Geometry: final body of the model. Coordinates: model frame, mm. A direction names the side the tool comes from. Give positions to 0.01 mm unless a question says otherwise; leave off trailing zeros. Write each loop counter-clockwise with the first axis right and the second up, starting at its lowest first coordinate (ties: lowest second). Pieces come first, ordered by that corner, then holes. Notation, with made-up numbers: (60.25, 45) -> (72.25, 45) arc R34 cw to (72.25, 81) -> close; hole circle Ø10 at (33.25, 53). An arc over 180 degrees is marked (long way). Answer as a JSON object with one key per item and string values.
from build123d import *

# Parameters (mm, degrees)
SKETCH001_W     = 40
SKETCH001_H     = 13.5
PAD_DEPTH       = 1
FILLET_R        = 2
SKETCH002_R     = 0.8
POCKET_DEPTH    = 85.45809
SKETCH_W        = 20
SKETCH_H        = 1.5
PAD001_DEPTH    = 3
SKETCH003_W     = 44
SKETCH003_H     = 1.5
PAD002_DEPTH    = 10
SKETCH005_R     = 2
POCKET001_DEPTH = 98.464305
PAD003_DEPTH    = 20


with BuildPart() as part:
    # Sketch001 → Pad (new body)
    with BuildSketch(Plane.XY):
        Rectangle(SKETCH001_W, SKETCH001_H)
    extrude(amount=PAD_DEPTH)

    # Fillet
    fillet_edges = [part.edges().sort_by_distance(p)[0] for p in [
        (20, 6.75, 0.5),
        (20, -6.75, 0.5),
        (-20, -6.75, 0.5),
        (-20, 6.75, 0.5),
    ]]
    fillet(fillet_edges, radius=FILLET_R)

    # Sketch002 (on Face5 of Fillet) → Pocket (cut, through all)
    with BuildSketch(Plane.XY.offset(1)):
        with Locations((-11, 5.75)):
            Circle(SKETCH002_R)
    pocket = extrude(amount=-POCKET_DEPTH, mode=Mode.SUBTRACT)

    # Mirrored: Pocket across Sketch002 V_Axis
    add(pocket.mirror(Plane(origin=(0, 0, 1), x_dir=(0, 0, 1), z_dir=(1, 0, 0))), mode=Mode.SUBTRACT)

    # Sketch (on Face5 of Mirrored) → Pad001 (join)
    with BuildSketch(Plane.XY.offset(1)):
        with Locations((0, -5.25)):
            Rectangle(SKETCH_W, SKETCH_H)
    extrude(amount=PAD001_DEPTH)

    # Sketch003 (on Face17 of Pad001) → Pad002 (join)
    with BuildSketch(Plane.XY.offset(4)):
        with Locations((0, -5.25)):
            Rectangle(SKETCH003_W, SKETCH003_H)
    extrude(amount=PAD002_DEPTH)

    # Sketch005 (on Face17 of Pad002) → Pocket001 (cut, through all)
    with BuildSketch(Plane(origin=(0, -4.5, 0), x_dir=(-1, 0, 0), z_dir=(0, 1, 0))):
        with Locations((-20.5, 9)):
            Circle(SKETCH005_R)
    pocket001 = extrude(amount=-POCKET001_DEPTH, mode=Mode.SUBTRACT)

    # Mirrored001: Pocket001 across Sketch005 V_Axis
    add(pocket001.mirror(Plane(origin=(0, -4.5, 0), x_dir=(0, 1, 0), z_dir=(-1, 0, 0))), mode=Mode.SUBTRACT)

    # Sketch006 (on Face16 of Mirrored001) → Pad003 (join)
    with BuildSketch(Plane(origin=(-10, 0, 0), x_dir=(0, -1, 0), z_dir=(-1, 0, 0))):
        Polygon((4.5, 4), (1.5, 1), (4.5, 1), align=None)
    extrude(amount=-PAD003_DEPTH)


solid = part.part
Q1. Cut plane A-A (x = 20.5). Return the cut outline in (y, z).
Values:
{"outline": "(-6, 4) -> (-4.5, 4) -> (-4.5, 7) -> (-6, 7) -> close; (-6, 11) -> (-4.5, 11) -> (-4.5, 14) -> (-6, 14) -> close"}
Q2. Set-up query: faces 1 (the flat face through (16, -5, 4)), 2 (the flat face through (0, -6, 7)), 3 (the cylindrical face through (-19.43, -6.15, 0.51)). Return all of +Z, -Z, +X, -X, +Y, -Y with unobstructed straight access to the full face (end or side cutting, diameter ignored); none if empty.
Values:
{"face 1": "+X, +Y, -Y", "face 2": "+Z, +X, -X, -Y", "face 3": "-Z, -X, -Y"}
Q3. Cut plane B-B (x = -11). Return the cut outline in (y, z).
Values:
{"outline": "(-6.75, 0) -> (4.95, 0) -> (4.95, 1) -> (-6.75, 1) -> close; (-6, 4) -> (-4.5, 4) -> (-4.5, 14) -> (-6, 14) -> close; (6.55, 0) -> (6.75, 0) -> (6.75, 1) -> (6.55, 1) -> close"}
Q4. Cut plane D-D (y = 5.75). Return the cut outline in (x, z), and give its area (3 significant figures).
Values:
{"outline": "(-19.73, 0) -> (-11.8, 0) -> (-11.8, 1) -> (-19.73, 1) -> close; (-10.2, 0) -> (10.2, 0) -> (10.2, 1) -> (-10.2, 1) -> close; (11.8, 0) -> (19.73, 0) -> (19.73, 1) -> (11.8, 1) -> close", "area": "36.3 mm²"}
Q5. Material intervals for L1, parallel to Z at x = -20.5, y = -5.3; L2, parallel to Y at x = -11, z = 0.6; L3, parallel to X at y = -5.6, z = 9, sorted ascending. Write a range as from..to.
Values:
{"L1": "4..7, 11..14", "L2": "-6.75..4.95, 6.55..6.75", "L3": "-18.5..18.5"}
Q6. Mould query, pull axis Z, two halves, no side actions, for faces 4 (the flat face through (-10, -4, 2)), 5 (the flat face through (10, -4, 2)), 6 (the cylindrical face through (-19.43, 6.15, 0.51)), 7 (the flat face through (0, -5, 14)). Classes: pulls with the +Z half, pulls with the -Z half, needs draft (parallel to the pull), parting line crosses it, or undercut.
Values:
{"face 4": "undercut", "face 5": "undercut", "face 6": "needs draft", "face 7": "pulls with the +Z half"}
Q7. Cut plane C-C (x = -4). Return the cut outline in (y, z), and give its area (3 significant figures).
Values:
{"outline": "(-6.75, 0) -> (6.75, 0) -> (6.75, 1) -> (-1.5, 1) -> (-4.5, 4) -> (-4.5, 14) -> (-6, 14) -> (-6, 1) -> (-6.75, 1) -> close", "area": "37.5 mm²"}
Q8. First-contact query: P1, Ø1.1, axis at y = 0, z = 0.5, coming from the -X side; P2, Ø3.5, axis at y = -3, z = 3, coming from the +X side; P3, Ø2.5, axis at y = -3, z = 3, coming from the -X side. Flat tips, straight axial feed; report the tip coordinate or a pass-through.
Values:
{"P1": "x = -20", "P2": "x = 10", "P3": "x = -10"}
